from build123d import *

# Parameters (mm, degrees)
ESQUISSE1_R             = 2
ESQUISSE1_R_2           = 1.65
ESQUISSE1_W             = 65
ESQUISSE1_H             = 35
ESQUISSE1_W_2           = 30
ESQUISSE1_H_2           = 5
ESQUISSE1_H_3           = 11
BOSS_EXTRU_1_DEPTH      = 3
ENL_V_MAT_EXTRU_1_DEPTH = 10


with BuildPart() as part:
    # Esquisse1 → Boss.-Extru.1 (new body)
    with BuildSketch(Plane.XY):
        Polygon((37.118802154, 168.871977627), (100.962812921, 58.290907218), (96.632685902, 55.790907218), (91.632685902, 64.451161256), (82.106406461, 58.951161256), (87.106406461, 50.290907218), (0, 0), (-87.106406461, 50.290907218), (-82.106406461, 58.951161256), (-91.632685902, 64.451161256), (-96.632685902, 55.790907218), (-100.962812921, 58.290907218), (-37.118802154, 168.871977627), align=None)
        with Locations((-84.369546181, 66.031288275)):
            Circle(ESQUISSE1_R, mode=Mode.SUBTRACT)
        with Locations((84.369546181, 66.031288275)):
            Circle(ESQUISSE1_R, mode=Mode.SUBTRACT)
        with Locations((-19, 97.371977627)):
            Circle(ESQUISSE1_R_2, mode=Mode.SUBTRACT)
        with Locations((19, 97.371977627)):
            Circle(ESQUISSE1_R_2, mode=Mode.SUBTRACT)
        with Locations((19, 158.371977627)):
            Circle(ESQUISSE1_R_2, mode=Mode.SUBTRACT)
        with Locations((-19, 158.371977627)):
            Circle(ESQUISSE1_R_2, mode=Mode.SUBTRACT)
        with Locations((-19, 59.371977627)):
            Circle(ESQUISSE1_R_2, mode=Mode.SUBTRACT)
        with Locations((0, 7.342924489)):
            Circle(ESQUISSE1_R, mode=Mode.SUBTRACT)
        with Locations((19, 59.371977627)):
            Circle(ESQUISSE1_R_2, mode=Mode.SUBTRACT)
        with Locations((19, 29.371977627)):
            Circle(ESQUISSE1_R_2, mode=Mode.SUBTRACT)
        with Locations((-19, 29.371977627)):
            Circle(ESQUISSE1_R_2, mode=Mode.SUBTRACT)
        with Locations((-45.775934694, 132.877384219)):
            Circle(ESQUISSE1_R, mode=Mode.SUBTRACT)
        with Locations((-60.775934694, 106.896622105)):
            Circle(ESQUISSE1_R, mode=Mode.SUBTRACT)
        with Locations((60.775934694, 106.896622105)):
            Circle(ESQUISSE1_R, mode=Mode.SUBTRACT)
        with Locations((45.775934694, 132.877384219)):
            Circle(ESQUISSE1_R, mode=Mode.SUBTRACT)
        with Locations((0, 130.371977627)):
            Rectangle(ESQUISSE1_W, ESQUISSE1_H, mode=Mode.SUBTRACT)
        with Locations((0, 59.371977627)):
            Rectangle(ESQUISSE1_W_2, ESQUISSE1_H_2, mode=Mode.SUBTRACT)
        with Locations((0, 29.371977627)):
            Rectangle(ESQUISSE1_W_2, ESQUISSE1_H_2, mode=Mode.SUBTRACT)
        with Locations((0, 97.371977627)):
            Rectangle(ESQUISSE1_W_2, ESQUISSE1_H_3, mode=Mode.SUBTRACT)
        Polygon((-53.039074415, 131.2972572), (-63.039074415, 113.976749124), (-54.378820377, 108.976749124), (-44.378820377, 126.2972572), align=None, mode=Mode.SUBTRACT)
        Polygon((63.039074415, 113.976749124), (54.378820377, 108.976749124), (44.378820377, 126.2972572), (53.039074415, 131.2972572), align=None, mode=Mode.SUBTRACT)
        with Locations((0, 158.371977627)):
            Rectangle(ESQUISSE1_W_2, ESQUISSE1_H_3, mode=Mode.SUBTRACT)
    extrude(amount=BOSS_EXTRU_1_DEPTH)

    # Esquisse2 → Enlèv. mat.-Extru.1 (cut)
    with BuildSketch(Plane(origin=(0, 0, 0), x_dir=(-1, 0, 0), z_dir=(0, 0, -1))):
        with BuildLine():
            Line((-45.427639482, 26.227659884), (-79.321398517, 45.796230786))
            ThreePointArc((-79.321398517, 45.796230786), (-52.612809671, 52.91972186), (-45.427639482, 26.227659884))
        make_face()
    extrude(amount=-ENL_V_MAT_EXTRU_1_DEPTH, mode=Mode.SUBTRACT)


solid = part.part
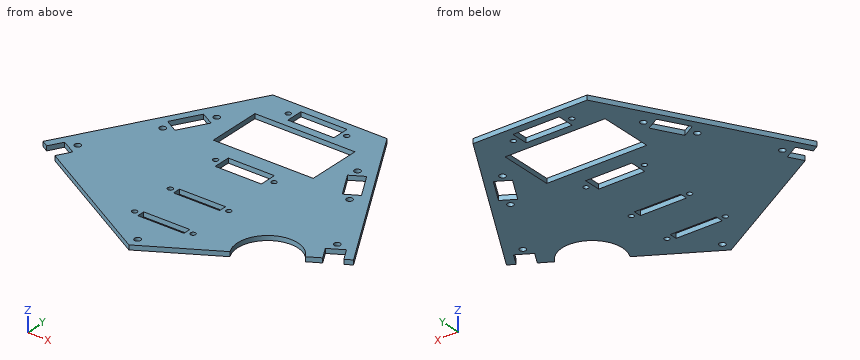
The model under review builds one solid part; all positions refer to its coordinate system, in mm. Coordinates: 2 decimals unless noted, no trailing zeros. Loops run counter-clockwise (first coordinate to the right, second up) from the corner with the lowest first, then second, coordinate; pieces in that order, holes last. Notation, with made-up numbers: (65.5, -0.75) -> (99.5, -0.75) arc R35 cw to (99.5, 33.25) -> close; hole circle Ø5 at (18.5, 69). An arc over 180 degrees is marked (long way). Use a Markdown table: item, result. Add a question column.
1. To check wall thickness, follow line 1 (X direction, y = 117, z = 2.05); line 2 (Y direction, x = 19, z = 1.5); line 3 (X direction, y = 28.5, z = 0.95). State the ranges of each line that lie inside material, in increasing order.
2. Add section A-A on x = -25. Write out the cut boundary in (y, z), plus the area to 3 significant figures.
3. Add section B-B on y = 138. Write out the cut boundary in (x, z), plus the area to 3 significant figures.
4. Clearance check with flat-ended pins moving along their axes: pin 1 Ø3 at (x, y) = (19, 29.37) entering from +Z; pin 2 Ø1.5 at (y, z) = (47, 0.5) entering from -X; pin 3 Ø0.9 at (x, z) = (-7, 1) entering from -Y; pin 4 Ø1.5 at (x, z) = (71.5, 2.5) entering from -Y. State where each tip first meets the part, or that it passes through.
5. Add section D-D on z = 1.1. Give the number of separate pieces and of enclosed holes in the cut face, plus the area to 3 significant figures.
6. Add section C-C on x = -4.5. Write out the cut boundary in (y, z), plus the area to 3 significant figures.
Returned:
| question | item | result |
|---|---|---|
| 1 | line 1 | x = -67.07 to -61.29, -49.75 to -32.5, 32.5 to 49.75, 61.29 to 67.07 |
| 1 | line 2 | y = 10.97 to 27.72, 31.02 to 57.72, 61.02 to 95.72, 99.02 to 112.87, 147.87 to 156.72, 160.02 to 168.87 |
| 1 | line 3 | x = -49.36 to -20.4, -17.6 to -15, 15 to 17.6, 20.4 to 44.31 |
| 2 | outline | (14.43, 0) -> (112.87, 0) -> (112.87, 3) -> (14.43, 3) -> close; (147.87, 0) -> (168.87, 0) -> (168.87, 3) -> (147.87, 3) -> close |
| 2 | area | 358 mm² |
| 3 | outline | (-54.94, 0) -> (-32.5, 0) -> (-32.5, 3) -> (-54.94, 3) -> close; (32.5, 0) -> (54.94, 0) -> (54.94, 3) -> (32.5, 3) -> close |
| 3 | area | 135 mm² |
| 4 | pin 1 | passes through |
| 4 | pin 2 | stops at x = -82.71 |
| 4 | pin 3 | stops at y = 3.78 |
| 4 | pin 4 | stops at y = 52.88 |
| 5 | separate pieces | 1 |
| 5 | enclosed holes | 22 |
| 5 | area | 16,500 mm² |
| 6 | outline | (2.6, 0) -> (26.87, 0) -> (26.87, 3) -> (2.6, 3) -> close; (31.87, 0) -> (56.87, 0) -> (56.87, 3) -> (31.87, 3) -> close; (61.87, 0) -> (91.87, 0) -> (91.87, 3) -> (61.87, 3) -> close; (102.87, 0) -> (112.87, 0) -> (112.87, 3) -> (102.87, 3) -> close; (147.87, 0) -> (152.87, 0) -> (152.87, 3) -> (147.87, 3) -> close; (163.87, 0) -> (168.87, 0) -> (168.87, 3) -> (163.87, 3) -> close |
| 6 | area | 298 mm² |
